The listing builds one solid part. Answer for the finished solid, in the listing's coordinates (mm). Coordinates: 2 decimals unless noted, no trailing zeros. Order: outer loops, then holes, each group sorted by start corner. A loop starts at its lowest first (then second) coordinate and runs counter-clockwise, first axis right, second up. Notation, with made-up numbers: (7, -18) - (15, -18) arc R12 ccw to (15, -13) - close; hole circle Ø9 at (-25, 70). An arc over 180 degrees is marked (long way). Use a Markdown table: item, result. Add a question column.
Item 1: Flat-ended cylindrical pins translate along their axes: P1, Ø8, axis at x = -4, y = -5, coming from the -Z side; P2, Ø1.5, axis at y = -9.5, z = 1.5, coming from the +X side. Find the tip coordinate at first contact, or state that the pin passes through.
Item 2: The part is cut by section B-B, the plane z = 0.9. Give the vertices of the cut face in (x, y), then the cut area to 3 significant figures.
Item 3: Find the intervals of material crossed by line 1 along X through (y, z) = (-10.75, 2.05); line 2 along X through (y, z) = (11, 0.25); line 3 along Y through (x, z) = (-0.5, 1.45), in increasing order.
from build123d import *

# Parameters (mm, degrees)
F0_W     = 32
F0_H     = 25
F1_DEPTH = 2.5
F2_R     = 2.5
F3_SIZE2 = 2.49999
F3_SIZE  = 1.750509


# Not quite as in the source:
# - a fillet or chamfer is up to 0.001 mm smaller than in the source, because OpenCascade refuses the exact size


with BuildPart() as f1:
    # F0 (on Top) → F1 (new body)
    with BuildSketch(Plane.XY):
        Rectangle(F0_W, F0_H)
    extrude(amount=F1_DEPTH)

    # F2
    f2_edges = [f1.edges().sort_by_distance(p)[0] for p in [
        (-16, -12.5, 1.25),
        (16, -12.5, 1.25),
        (16, 12.5, 1.25),
        (-16, 12.5, 1.25),
    ]]
    fillet(f2_edges, radius=F2_R)

    # F3 (size 1.7505188455 and 2.5 in the source; OpenCascade refuses exactly that, so slightly less here)
    f3_edges = [f1.edges().sort_by_distance(p)[0] for p in [
        (0, -12.5, 2.5),
        (-16, 0, 2.5),
        (15.267767, -11.767767, 2.5),
        (16, 0, 2.5),
        (15.267767, 11.767767, 2.5),
        (0, 12.5, 2.5),
        (-15.267767, 11.767767, 2.5),
        (-15.267767, -11.767767, 2.5),
    ]]
    f3_side = f1.faces().sort_by_distance((0, 0, 2.5))[0]
    chamfer(f3_edges, length=F3_SIZE, length2=F3_SIZE2, reference=f3_side)


solid = f1.part
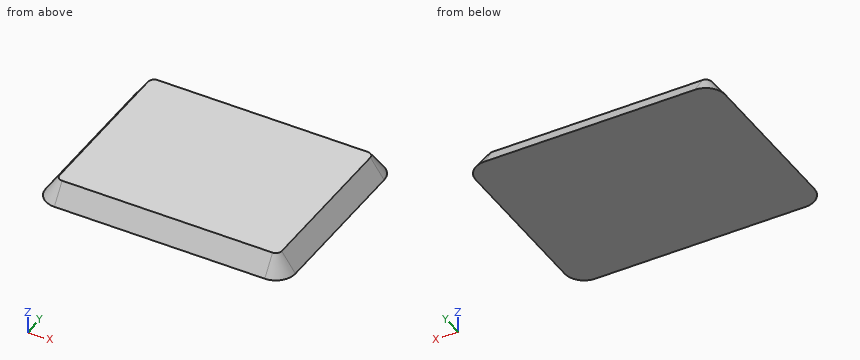
Solution:
| question | item | result |
|---|---|---|
| 1 | P1 | stops at z = 0 |
| 1 | P2 | stops at x = 15.47 |
| 2 | outline | (-15.37, -10) arc R1.87 ccw to (-13.5, -11.87) - (13.5, -11.87) arc R1.87 ccw to (15.37, -10) - (15.37, 10) arc R1.87 ccw to (13.5, 11.87) - (-13.5, 11.87) arc R1.87 ccw to (-15.37, 10) - close |
| 2 | area | 727 mm2 |
| 3 | line 1 | x = -14.26 to 14.26 |
| 3 | line 2 | x = -15.6 to 15.6 |
| 3 | line 3 | y = -11.48 to 11.48 |
